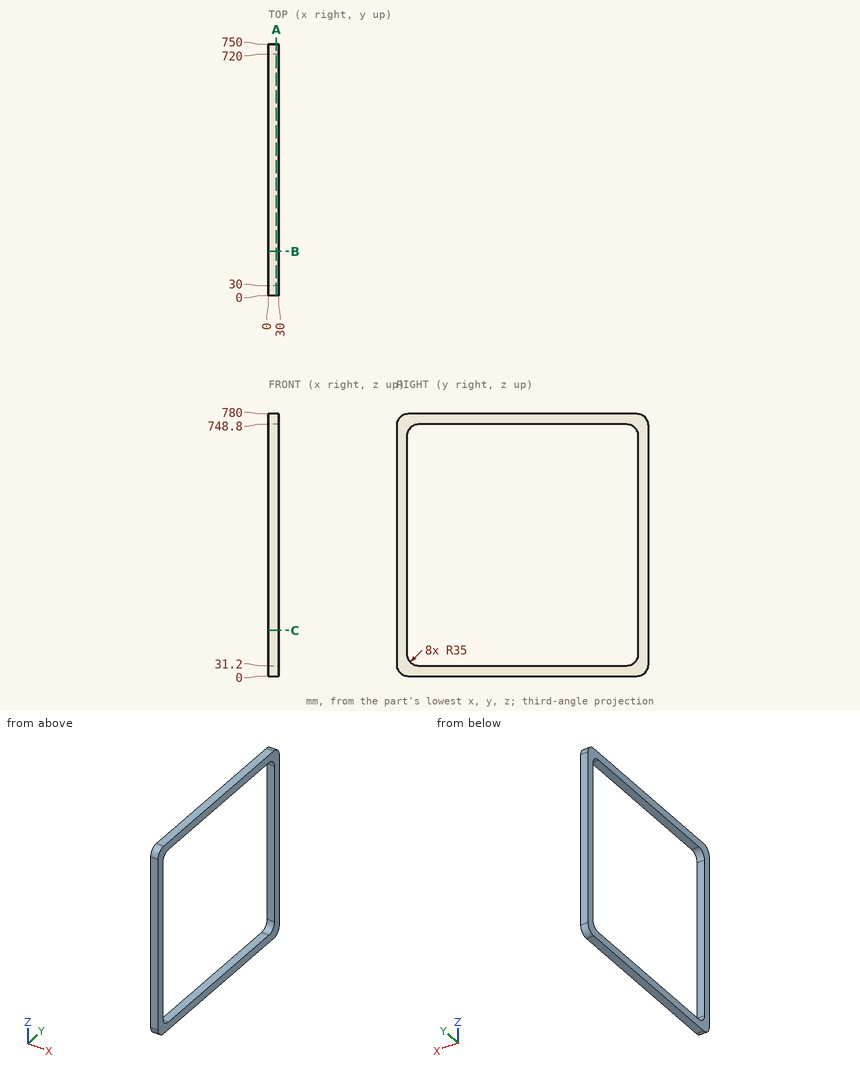
Design review of the part shown in the three views and the two pictorial views. Dimensions are in mm from the part's minimum x, y and z. Round coordinates to 2 decimals unless told otherwise and drop trailing zeros. Loops run counter-clockwise (first coordinate to the right, second up) from the corner with the lowest first, then second, coordinate; pieces in that order, holes last.
1) Consider section A-A on x = 23.5. State the section outline as (y, z) points, then the cut area to 3 significant figures.
Values follow:
outline: (0, 35) arc R35 ccw to (35, 0) - (715, 0) arc R35 ccw to (750, 35) - (750, 745) arc R35 ccw to (715, 780) - (35, 780) arc R35 ccw to (0, 745) - close; hole (30, 66.2) arc R35 ccw to (65, 31.2) - (685, 31.2) arc R35 ccw to (720, 66.2) - (720, 713.8) arc R35 ccw to (685, 748.8) - (65, 748.8) arc R35 ccw to (30, 713.8) - close
area: 89,900 mm2
2) Consider section C-C on z = 135.5. State the section outline as (x, y) points, then the cut area to 3 significant figures.
Values follow:
outline: (0, 0) - (30, 0) - (30, 30) - (0, 30) - close; (0, 720) - (30, 720) - (30, 750) - (0, 750) - close
area: 1,800 mm2
3) Consider section B-B on y = 132.5. State the section outline as (x, z) points, then the cut area to 3 significant figures.
Values follow:
outline: (0, 0) - (30, 0) - (30, 31.2) - (0, 31.2) - close; (0, 748.8) - (30, 748.8) - (30, 780) - (0, 780) - close
area: 1,870 mm2
4) Wall thickness on line 1 along Y through (x, z) = (6.25, 413); line 2 along Z through (x, y) = (9.75, 155); line 3 along Z through (x, y) = (1.75, 708): over which ranges is each line inside the solid? List them lowest first.
Values follow:
line 1: y = 0 to 30, 720 to 750
line 2: z = 0 to 31.2, 748.8 to 780
line 3: z = 0 to 39.82, 740.18 to 780
